CAD build for the part. Positions are in the model's coordinates, mm. A direction names the side the tool comes from. Give positions to 0.01 mm unless a question says otherwise; leave off trailing zeros. Loops run counter-clockwise (first coordinate to the right, second up) from the corner with the lowest first, then second, coordinate; pieces in that order, holes last.
```python
from build123d import *

# Parameters (mm, degrees)
F0_W     = 100
F0_H     = 100
F1_DEPTH = 300
F2_W     = 30
F2_H     = 35
F2_W_2   = 35
F2_H_2   = 30
F3_DEPTH = 100


with BuildPart() as f1:
    # F0 (on Top) → F1 (new body)
    with BuildSketch(Plane.XY):
        Rectangle(F0_W, F0_H)
    extrude(amount=F1_DEPTH)

    # F2 (on face) → F3 (join)
    with BuildSketch(Plane.XY.offset(300)):
        with Locations((0, 32.5)):
            Rectangle(F2_W, F2_H)
        with Locations((32.5, 0)):
            Rectangle(F2_W_2, F2_H_2)
        Rectangle(F2_W, F2_H_2)
        with Locations((-32.5, 0)):
            Rectangle(F2_W_2, F2_H_2)
        with Locations((0, -32.5)):
            Rectangle(F2_W, F2_H)
    extrude(amount=F3_DEPTH)


solid = f1.part
```
1. Probe line 1 along X through (y, z) = (-29, 351.5); line 2 along Z through (x, y) = (27, 34). List the from-to ranges inside material, lowest first.
Responses:
line 1: x = -15 to 15
line 2: z = 0 to 300
2. Saw through at A-A, the plane y = -43. List the corners of the cut face in (x, z), and give its area (3 significant figures).
Responses:
outline: (-50, 0) - (50, 0) - (50, 300) - (15, 300) - (15, 400) - (-15, 400) - (-15, 300) - (-50, 300) - close
area: 33,000 mm2
3. Tool access for faces 1 (the face through (-33, 33, 300)), 2 (the face through (15, -33, 349)), 3 (the face through (-1, 1, 0)), 4 (the face through (15, 32, 349)), 5 (the face through (-33, -15, 349)): list every direction of +Z, -Z, +X, -X, +Y, -Y with a clear straight run to the whole face (end or side of a thin tool).
Responses:
face 1: +Z, -X, +Y
face 2: +Z, +X, -Y
face 3: -Z, +X, -X, +Y, -Y
face 4: +Z, +X, +Y
face 5: +Z, -X, -Y
4. Drop flat-ended pins along their axis: pin 1 (17.5 mm diameter, centred on y = -33, z = 325, fed in from -X); pin 2 (6 mm diameter, centred on x = -34, y = -27, fed in from +Z); pin 3 (17.5 mm diameter, centred on y = -26.5, z = 362, fed in from +X); pin 4 (5 mm diameter, centred on x = 29.5, y = 0, fed in from -Z). Give the stop position or say it passes through.
Responses:
pin 1: stops at x = -15
pin 2: stops at z = 300
pin 3: stops at x = 15
pin 4: stops at z = 0
